from build123d import *
from build123d.topology import SkipClean

# Parameters (mm, degrees)
SKETCH2_W           = 108
SKETCH2_H           = 72
BOSS_EXTRUDE1_DEPTH = 20.64
SHELL1_T            = 5
SKETCH3_W           = 118
SKETCH3_H           = 82
CUT_EXTRUDE1_DEPTH  = 3
FILLET1_R           = 10
SKETCH13_W          = 16.51
SKETCH13_H          = 14.478
SKETCH13_R          = 3.249999977
BOSS_EXTRUDE4_DEPTH = 3.175
BOSS_EXTRUDE2_DEPTH = 8.255
CUT_EXTRUDE4_DEPTH  = 6.35
CUT_EXTRUDE2_DEPTH  = 1.875
FILLET3_R           = 2.38
FILLET4_R           = 4.92
FILLET5_R           = 2.38


with BuildPart() as part:
    # Sketch2 → Boss-Extrude1 (new body)
    with BuildSketch(Plane.XY):
        Rectangle(SKETCH2_W, SKETCH2_H)
    extrude(amount=BOSS_EXTRUDE1_DEPTH)

    # Shell1
    shell1_openings = [part.faces().sort_by_distance(p)[0] for p in [
        (0, 0, 20.64),
    ]]
    offset(amount=SHELL1_T, openings=shell1_openings, kind=Kind.INTERSECTION)

    # Sketch3 → Cut-Extrude1 (cut)
    with BuildSketch(Plane(origin=(0, 0, -5), x_dir=(-1, 0, 0), z_dir=(0, 0, -1))):
        Rectangle(SKETCH3_W, SKETCH3_H)
    extrude(amount=-CUT_EXTRUDE1_DEPTH, mode=Mode.SUBTRACT)

    # Fillet1
    fillet1_edges = [part.edges().sort_by_distance(p)[0] for p in [
        (54, -36, 10.32),
        (54, 36, 10.32),
        (-54, 36, 10.32),
        (-54, -36, 10.32),
    ]]
    fillet(fillet1_edges, radius=FILLET1_R)

    # Sketch13 → Boss-Extrude4 (add)
    with BuildSketch(Plane(origin=(0, 41, 0), x_dir=(1, 0, 0), z_dir=(0, 1, 0))):
        with Locations((-67.255, -5.239)):
            Rectangle(SKETCH13_W, SKETCH13_H)
        with Locations((-69.16, -5.239)):
            Circle(SKETCH13_R, mode=Mode.SUBTRACT)
    boss_extrude4 = extrude(amount=-BOSS_EXTRUDE4_DEPTH)

    # Mirror4: Boss-Extrude4 across plane
    add(boss_extrude4.mirror(Plane(origin=(0, 0, 0), x_dir=(0, 0, 1), z_dir=(1, 0, 0))))

    # Sketch6 → Boss-Extrude2 (add)
    with BuildSketch(Plane.XY.offset(20.64)):
        with BuildLine():
            Line((59, -41), (60.27, -41))
            ThreePointArc((60.27, -41), (65.732714697, -34.86066586), (59, -30.148635688))
            Line((59, -30.148635688), (59, -41))
        make_face()
        with BuildLine():
            ThreePointArc((59, 30.148635688), (65.77, 35.5), (59, 40.851364312))
            Line((59, 40.851364312), (59, 30.148635688))
        make_face()
        with BuildLine():
            ThreePointArc((-59, -30.148635688), (-65.77, -35.5), (-59, -40.851364312))
            Line((-59, -40.851364312), (-59, -30.148635688))
        make_face()
        with BuildLine():
            ThreePointArc((-59, 40.851364312), (-65.77, 35.5), (-59, 30.148635688))
            Line((-59, 30.148635688), (-59, 40.851364312))
        make_face()
    boss_extrude2 = extrude(amount=-BOSS_EXTRUDE2_DEPTH)

    # Sketch6<4> → Cut-Extrude4 (cut)
    with BuildSketch(Plane.XY.offset(20.64)):
        with BuildLine():
            Line((59, 38.245491759), (59, 32.754508241))
            ThreePointArc((59, 32.754508241), (61.899244457, 32.951238046), (63.295, 35.5))
            ThreePointArc((63.295, 35.5), (61.899244457, 38.048761954), (59, 38.245491759))
        make_face()
        with BuildLine():
            ThreePointArc((59, 38.245491759), (57.245, 35.5), (59, 32.754508241))
            Line((59, 32.754508241), (59, 38.245491759))
        make_face()
        with BuildLine():
            Line((59, -38.245491759), (59, -32.754508241))
            ThreePointArc((59, -32.754508241), (57.245, -35.5), (59, -38.245491759))
        make_face()
        with BuildLine():
            ThreePointArc((63.295, -35.5), (61.899244457, -32.951238046), (59, -32.754508241))
            Line((59, -32.754508241), (59, -38.245491759))
            ThreePointArc((59, -38.245491759), (61.899244457, -38.048761954), (63.295, -35.5))
        make_face()
        with BuildLine():
            ThreePointArc((-59, -38.245491759), (-57.721238046, -37.129244457), (-57.245, -35.5))
            ThreePointArc((-57.245, -35.5), (-57.721238046, -33.870755543), (-59, -32.754508241))
            Line((-59, -32.754508241), (-59, -38.245491759))
        make_face()
        with BuildLine():
            Line((-59, -38.245491759), (-59, -32.754508241))
            ThreePointArc((-59, -32.754508241), (-63.295, -35.5), (-59, -38.245491759))
        make_face()
        with BuildLine():
            Line((-59, 38.245491759), (-59, 32.754508241))
            ThreePointArc((-59, 32.754508241), (-57.721238046, 33.870755543), (-57.245, 35.5))
            ThreePointArc((-57.245, 35.5), (-57.721238046, 37.129244457), (-59, 38.245491759))
        make_face()
        with BuildLine():
            ThreePointArc((-59, 38.245491759), (-63.295, 35.5), (-59, 32.754508241))
            Line((-59, 32.754508241), (-59, 38.245491759))
        make_face()
    cut_extrude4 = extrude(amount=-CUT_EXTRUDE4_DEPTH, mode=Mode.SUBTRACT)

    # Mirror5: Boss-Extrude2, Cut-Extrude4 across plane
    with SkipClean():  # the faces are left unmerged after this step: merging them gives an invalid solid
        add(boss_extrude2.mirror(Plane(origin=(0, 0, 0), x_dir=(0, 0, 1), z_dir=(1, 0, 0))))
        add(cut_extrude4.mirror(Plane(origin=(0, 0, 0), x_dir=(0, 0, 1), z_dir=(1, 0, 0))), mode=Mode.SUBTRACT)

    # Sketch5 → Cut-Extrude2 (cut)
    with SkipClean():  # the faces are left unmerged after this step: merging them gives an invalid solid
        with BuildSketch(Plane.XY.offset(20.64)):
            with BuildLine():
                Line((46.071067812, -39.11), (-46.071067812, -39.11))
                ThreePointArc((-46.071067812, -39.11), (-54.050767838, -35.804700026), (-57.356067812, -27.825))
                Line((-57.356067812, -27.825), (-57.356067812, 28.071067812))
                ThreePointArc((-57.356067812, 28.071067812), (-54.050767838, 36.050767838), (-46.071067812, 39.356067812))
                Line((-46.071067812, 39.356067812), (46.071067812, 39.356067812))
                ThreePointArc((46.071067812, 39.356067812), (54.050767838, 36.050767838), (57.356067812, 28.071067812))
                Line((57.356067812, 28.071067812), (57.356067812, -27.825))
                ThreePointArc((57.356067812, -27.825), (54.050767838, -35.804700026), (46.071067812, -39.11))
            make_face()
            with BuildLine():
                Line((46.071067812, -36.54), (-46.071067812, -36.54))
                ThreePointArc((-46.071067812, -36.54), (-52.23350341, -33.987435598), (-54.786067812, -27.825))
                Line((-54.786067812, -27.825), (-54.786067812, 28.071067812))
                ThreePointArc((-54.786067812, 28.071067812), (-52.23350341, 34.23350341), (-46.071067812, 36.786067812))
                Line((-46.071067812, 36.786067812), (46.071067812, 36.786067812))
                ThreePointArc((46.071067812, 36.786067812), (52.23350341, 34.23350341), (54.786067812, 28.071067812))
                Line((54.786067812, 28.071067812), (54.786067812, -27.825))
                ThreePointArc((54.786067812, -27.825), (52.23350341, -33.987435598), (46.071067812, -36.54))
            make_face(mode=Mode.SUBTRACT)
        extrude(amount=-CUT_EXTRUDE2_DEPTH, mode=Mode.SUBTRACT)

    # Fillet3
    fillet3_edges = [part.edges().sort_by_distance(p)[0] for p in [
        (59, -30.148635688, 16.5125),
        (-65.254413205, 37.825, 12.4315),
        (-59, 30.148635688, 16.5125),
        (-59, -30.148635688, 16.5125),
        (65.254413205, 37.825, 12.4315),
        (59, 30.148635688, 16.5125),
    ]]
    fillet(fillet3_edges, radius=FILLET3_R)

    # Fillet4
    fillet4_edges = [part.edges().sort_by_distance(p)[0] for p in [
        (59, -41, 5.1925),
        (-59, -41, 5.1925),
        (-59, 37.825, 5.1925),
        (59, 37.825, 5.1925),
    ]]
    fillet(fillet4_edges, radius=FILLET4_R)

    # Fillet5
    fillet5_edges = [part.edges().sort_by_distance(p)[0] for p in [
        (-75.51, 39.4125, 12.478),
        (-75.51, 39.4125, -2),
        (75.51, 39.4125, -2),
        (75.51, 39.4125, 12.478),
    ]]
    fillet(fillet5_edges, radius=FILLET5_R)


solid = part.part
Can you work these out from the model? Positions are in its coordinate system, mm. A direction names the side the tool comes from. Coordinates: 2 decimals unless noted, no trailing zeros. Loops run counter-clockwise (first coordinate to the right, second up) from the corner with the lowest first, then second, coordinate; pieces in that order, holes last. Notation, with made-up numbers: M 37.25,15.5 L 93.25,15.5 A32 cw 93.25,41.5 Z; hole C 38.25,53.25 d2. An arc over 180 degrees is marked long. Return JSON: item names as keys, results as strings. Group by question number.
Item 1: If I drill on L1, parallel to Y at x = 22, z = 2.25; L2, parallel to X at y = -26, z = 15; L3, parallel to Y at x = 60.27, z = 19 (3 decimals), over which ranges is the centre line in solid material (lowest first)? Write a range as from..to.
Item 2: Imagine slicing it at B-B (y = -8). Please give me the cut outline in (x, z) (3 decimals).
Item 3: On a 3-axis mill with a long thin cutter (end or side, diameter ignored), from which of +Z, -Z, +X, -X, +Y, -Y can I reach the whole of each face in a straight line? I mean faces 5 (the flat face through (-72.4, 37.825, 3.5)), 6 (the cylindrical face through (54, 36.1, 19.7)), 7 (the flat face through (-68, 40, 12.478)), 8 (the cylindrical face through (57.6, -39.52, 5.29)). Say none if no direction works.
Item 4: Thinking about a two-plate mould opening in X: for faces 1 (the cylindrical face through (-52.17, -34.05, 19.72)), 2 (the cylindrical face through (65.747, -36.003, 16.57)), 3 (the flat face through (1, 1, -2)), 4 (the cylindrical face through (66.06, 39.43, 4.26)), which applies, released by +X, released by -X, zero draft, split by the parting line, or undercut?
Item 5: Imagine slicing it at A-A (x = 26.5). Please give me the cut outline in (y, z) (3 decimals), and give its area (3 significant figures).
Item 6: I'm going to push flat-ended pins straight in: pin 1 Ø6 at (x, z) = (69.5, 2.5) entering from -Y (3 decimals); pin 2 Ø1.5 at (x, y) = (45, -27.5) entering from +Z; pin 3 Ø0.6 at (y, z) = (3.5, 19.5) entering from -X. Where does each tip first touch, or does it pass through?
Verdict:
{
 "1": {"L1": "y = -41..-36, 36..41", "L2": "x = -59..-54, 54..59", "L3": "y = -41..-38.525, -32.475..-29.804, 29.804..32.475, 38.525..41"},
 "2": {"outline": "M -59,-2 L 59,-2 L 59,20.64 L 57.356,20.64 L 57.356,18.765 L 54.786,18.765 L 54.786,20.64 L 54,20.64 L 54,0 L -54,0 L -54,20.64 L -54.786,20.64 L -54.786,18.765 L -57.356,18.765 L -57.356,20.64 L -59,20.64 Z"},
 "3": {"face 5": "-Z, -X, -Y", "face 6": "+Z", "face 7": "+Z, -X, +Y", "face 8": "-Z, +X, -Y"},
 "4": {"face 1": "undercut", "face 2": "released by +X", "face 3": "zero draft", "face 4": "undercut"},
 "5": {"outline": "M -41,-2 L 41,-2 L 41,20.64 L 39.356,20.64 L 39.356,18.765 L 36.786,18.765 L 36.786,20.64 L 36,20.64 L 36,0 L -36,0 L -36,20.64 L -36.54,20.64 L -36.54,18.765 L -39.11,18.765 L -39.11,20.64 L -41,20.64 Z", "area": "361 mm^2"},
 "6": {"pin 1": "stops at y = 37.825", "pin 2": "stops at z = 0", "pin 3": "stops at x = -59"}
}
